For this review, use the dimensioned drawing (mm, ordinates from the lowest corner) and the shaded views. A direction names the side the tool comes from. Round coordinates to 2 decimals unless told otherwise and drop trailing zeros. Write each loop counter-clockwise with the first axis right and the second up, starting at its lowest first coordinate (ties: lowest second). Pieces come first, ordered by that corner, then holes.
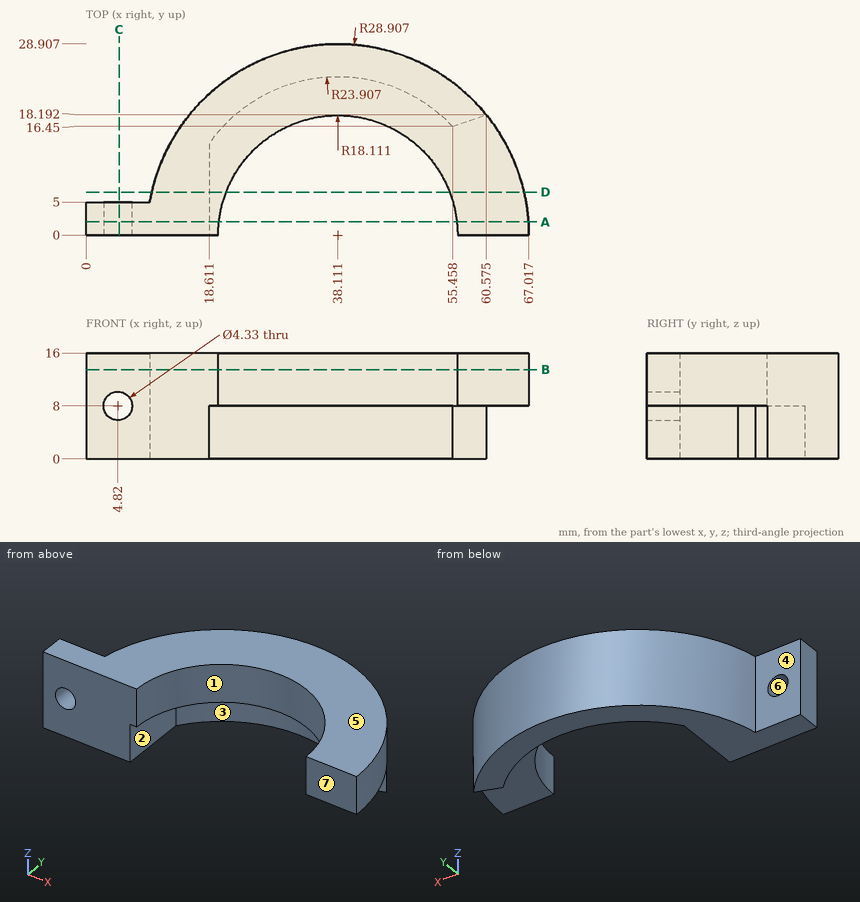
(1) We need section A-A, the plane y = 2. Give the boundary of the cut face in (x, z) (1 decimal), and give its area (3 significant figures).
Geometry check:
outline: (0, 0) - (18.6, 0) - (18.6, 8) - (20.1, 8) - (20.1, 16) - (0, 16) - close; (56.1, 8) - (66.9, 8) - (66.9, 16) - (56.1, 16) - close; hole circle Ø4.3 at (4.8, 8)
area: 382 mm2
(2) Mouldability with a two-part tool opening along Z and no side actions: class the marked faces 5, 6 and 7 as pulls with the +Z half, pulls with the -Z half, needs draft (parallel to the pull), parting line crosses it, or undercut.
Geometry check:
face 5: pulls with the +Z half
face 6: undercut
face 7: needs draft
(3) For the marked faces 1, 2, 3 and 4, list the 3-axis set-ups (+Z, -Z, +X, -X, +Y, -Y) from which the entire face can be reached by the end or side of a thin tool; tool diameter is ignored.
Geometry check:
face 1: +Z, -Z, -Y
face 2: -Z, +X, -Y
face 3: -Z, -Y
face 4: +Z, -Z, -X, +Y
(4) We need section B-B, the plane z = 13.5. Give the boundary of the cut face in (x, y), and give its area (3 significant figures).
Geometry check:
outline: (0, 0) - (20, 0) arc R18.11 cw to (56.22, 0) - (67.02, 0) arc R28.91 ccw to (9.64, 5) - (0, 5) - close
area: 844 mm2
(5) For line 1 along Y through (x, z) = (3.5, 6.25); line 2 along X through (y, z) = (16, 11.75) (1 decimal); line 3 along Z through (x, y) = (6, 4) (1 decimal), list the stretches that pass through material, from the lowest coordinate up.
Geometry check:
line 1: y = 0 to 5
line 2: x = 14 to 29.6, 46.6 to 62.2
line 3: z = 0 to 6.2, 9.8 to 16
(6) We need section C-C, the plane x = 5. Give the boundary of the cut face in (y, z).
Geometry check:
outline: (0, 0) - (5, 0) - (5, 5.84) - (0, 5.84) - close; (0, 10.16) - (5, 10.16) - (5, 16) - (0, 16) - close
(7) We need section D-D, the plane y = 6.5. Give the boundary of the cut face in (x, z) (1 decimal).
Geometry check:
outline: (9.9, 0) - (18.6, 0) - (18.6, 8) - (21.2, 8) - (21.2, 16) - (9.9, 16) - close; (55, 8) - (66.3, 8) - (66.3, 16) - (55, 16) - close
(8) For pin 1 Ø5 at (x, z) = (58.5, 3) entering from -Y (1 decimal); pin 2 Ø6 at (x, y) = (23, 3) entering from +Z; pin 3 Ø2 at (y, z) = (7.5, 7.5) entering from -X; pin 4 Ø4 at (x, z) = (56, 6.5) entering from +Y, all flat-tipped, find the tip position at first contact; note any pin that passes through.
Geometry check:
pin 1: stops at y = 16.6
pin 2: stops at z = 16
pin 3: stops at x = 9.94
pin 4: stops at y = 24.15
